Here's how the part is built. I have some questions about the finished solid (model axes, mm). A direction names the side the tool comes from. Coordinates: 2 decimals unless noted, no trailing zeros. Order: outer loops, then holes, each group sorted by start corner. A loop starts at its lowest first (then second) coordinate and runs counter-clockwise, first axis right, second up.
```python
from build123d import *

# Parameters (mm, degrees)
SKETCH_1_W                         = 1000
SKETCH_1_H                         = 368
SM_BASE_FLANGE_1_DEPTH             = 1
OTHER_START                        = -134.5
OTHER_1_DEPTH                      = 269
OTHER_1_2_DEPTH                    = 0.5
OTHER_START_2                      = 134
OTHER_1_3_DEPTH                    = 0.5
OTHER_START_3                      = -134
OTHER_1_4_DEPTH                    = 268
OTHER_START_4                      = -450.5
OTHER_2_DEPTH                      = 901
OTHER_2_2_DEPTH                    = 0.5
OTHER_START_5                      = 450
OTHER_2_3_DEPTH                    = 0.5
OTHER_START_6                      = -450
OTHER_2_4_DEPTH                    = 900
SM_EDGE_FLANGE_1_STRIP_W           = 5.4732
SM_EDGE_FLANGE_1_STRIP_H           = 1
SM_EDGE_FLANGE_1_STRIP_CUT_DEPTH   = 900
SM_EDGE_FLANGE_1_RELIEF_W          = 5.9732
SM_EDGE_FLANGE_1_RELIEF_H          = 0.5
SM_EDGE_FLANGE_1_RELIEF_CUT_DEPTH  = 1
SM_EDGE_FLANGE_1_DEPTH             = 900
SM_EDGE_FLANGE_1_FLAT_DEPTH        = 1
SM_EDGE_FLANGE_2_STRIP_W           = 5.4732
SM_EDGE_FLANGE_2_STRIP_H           = 1
SM_EDGE_FLANGE_2_STRIP_CUT_DEPTH   = 214.5
SM_EDGE_FLANGE_2_STRIP_2_W         = 5.4732
SM_EDGE_FLANGE_2_STRIP_2_H         = 1
SM_EDGE_FLANGE_2_STRIP_CUT_2_DEPTH = 412
SM_EDGE_FLANGE_2_STRIP_3_W         = 5.4732
SM_EDGE_FLANGE_2_STRIP_3_H         = 1
SM_EDGE_FLANGE_2_STRIP_CUT_3_DEPTH = 213.5
SM_EDGE_FLANGE_2_DEPTH             = 214.5
SM_EDGE_FLANGE_2_BEND_DEPTH        = 412
SM_EDGE_FLANGE_2_BEND_2_DEPTH      = 213.5
SKETCH_19_R                        = 3
CUT_EXTRUDE_1_DEPTH                = 534.120061525


# Read off the part's stored shape, not the designer's step: 斜接法兰1, 斜接法兰2
# Sheet-metal steps are written as plain solids
with BuildPart() as part:
    # Sketch 1 → 基体-法兰1 (new body)
    with BuildSketch(Plane.XY):
        Rectangle(SKETCH_1_W, SKETCH_1_H)
    extrude(amount=-SM_BASE_FLANGE_1_DEPTH)

    # Other 1 outline → Other 1 (cut)
    with BuildSketch(Plane(origin=(0, 0, 0), x_dir=(1, 0, 0), z_dir=(0, 1, 0)).offset(OTHER_START)):
        with BuildLine():
            Line((500, 1), (499.83604109, 1))
            ThreePointArc((499.83604109, 1), (499.195226164, 0.271171885), (498.2634, 0))
            Line((498.2634, 0), (500, 0))
            Line((500, 0), (500, 1))
        make_face()
    other_1 = extrude(amount=OTHER_1_DEPTH, mode=Mode.SUBTRACT)

    # Other 1 2 outline → Other 1 2 (cut)
    with BuildSketch(Plane(origin=(0, 0, 0), x_dir=(1, 0, 0), z_dir=(0, 1, 0)).offset(OTHER_START)):
        with BuildLine():
            ThreePointArc((498.2634, 0), (499.195226164, 0.271171885), (499.83604109, 1))
            Line((499.83604109, 1), (497.7634, 1))
            Line((497.7634, 1), (497.7634, 0))
            Line((497.7634, 0), (498.2634, 0))
        make_face()
    other_1_2 = extrude(amount=OTHER_1_2_DEPTH, mode=Mode.SUBTRACT)

    # Other 1 3 outline → Other 1 3 (cut)
    with BuildSketch(Plane(origin=(0, 0, 0), x_dir=(1, 0, 0), z_dir=(0, 1, 0)).offset(OTHER_START_2)):
        with BuildLine():
            ThreePointArc((498.2634, 0), (499.195226164, 0.271171885), (499.83604109, 1))
            Line((499.83604109, 1), (497.7634, 1))
            Line((497.7634, 1), (497.7634, 0))
            Line((497.7634, 0), (498.2634, 0))
        make_face()
    other_1_3 = extrude(amount=OTHER_1_3_DEPTH, mode=Mode.SUBTRACT)

    # Other 1 4 outline → Other 1 4 (add)
    with BuildSketch(Plane(origin=(0, 0, 0), x_dir=(1, 0, 0), z_dir=(0, 1, 0)).offset(OTHER_START_3)):
        with BuildLine():
            Line((500, 1.7366), (500, 18.2634))
            ThreePointArc((500, 18.2634), (499.491361636, 19.491361636), (498.2634, 20))
            Line((498.2634, 20), (485, 20))
            Line((485, 20), (485, 19))
            Line((485, 19), (498.2634, 19))
            ThreePointArc((498.2634, 19), (498.784254855, 18.784254855), (499, 18.2634))
            Line((499, 18.2634), (499, 1.7366))
            ThreePointArc((499, 1.7366), (498.784254855, 1.215745145), (498.2634, 1))
            Line((498.2634, 1), (499.83604109, 1))
            ThreePointArc((499.83604109, 1), (499.958514757, 1.359286442), (500, 1.7366))
        make_face()
    other_1_4 = extrude(amount=OTHER_1_4_DEPTH)

    # Other 2 outline → Other 2 (cut)
    with BuildSketch(Plane.YZ.offset(OTHER_START_4)):
        with BuildLine():
            ThreePointArc((182.2634, 0), (183.195226164, -0.271171885), (183.83604109, -1))
            Line((183.83604109, -1), (184, -1))
            Line((184, -1), (184, 0))
            Line((184, 0), (182.2634, 0))
        make_face()
    extrude(amount=OTHER_2_DEPTH, mode=Mode.SUBTRACT)

    # Other 2 2 outline → Other 2 2 (cut)
    with BuildSketch(Plane.YZ.offset(OTHER_START_4)):
        with BuildLine():
            Line((181.7634, -1), (183.83604109, -1))
            ThreePointArc((183.83604109, -1), (183.195226164, -0.271171885), (182.2634, 0))
            Line((182.2634, 0), (181.7634, 0))
            Line((181.7634, 0), (181.7634, -1))
        make_face()
    extrude(amount=OTHER_2_2_DEPTH, mode=Mode.SUBTRACT)

    # Other 2 3 outline → Other 2 3 (cut)
    with BuildSketch(Plane.YZ.offset(OTHER_START_5)):
        with BuildLine():
            Line((181.7634, -1), (183.83604109, -1))
            ThreePointArc((183.83604109, -1), (183.195226164, -0.271171885), (182.2634, 0))
            Line((182.2634, 0), (181.7634, 0))
            Line((181.7634, 0), (181.7634, -1))
        make_face()
    extrude(amount=OTHER_2_3_DEPTH, mode=Mode.SUBTRACT)

    # Other 2 4 outline → Other 2 4 (add)
    with BuildSketch(Plane.YZ.offset(OTHER_START_6)):
        with BuildLine():
            Line((184, -18.2634), (184, -1.7366))
            ThreePointArc((184, -1.7366), (183.958514757, -1.359286442), (183.83604109, -1))
            Line((183.83604109, -1), (182.2634, -1))
            ThreePointArc((182.2634, -1), (182.784254855, -1.215745145), (183, -1.7366))
            Line((183, -1.7366), (183, -18.2634))
            ThreePointArc((183, -18.2634), (182.784254855, -18.784254855), (182.2634, -19))
            Line((182.2634, -19), (169, -19))
            Line((169, -19), (169, -20))
            Line((169, -20), (182.2634, -20))
            ThreePointArc((182.2634, -20), (183.491361636, -19.491361636), (184, -18.2634))
        make_face()
    extrude(amount=OTHER_2_4_DEPTH)

    # 镜向1: Other 1, Other 1 2, Other 1 3, Other 1 4 across plane
    add(other_1.mirror(Plane(origin=(0, 0, 0), x_dir=(0, 0, 1), z_dir=(1, 0, 0))), mode=Mode.SUBTRACT)
    add(other_1_2.mirror(Plane(origin=(0, 0, 0), x_dir=(0, 0, 1), z_dir=(1, 0, 0))), mode=Mode.SUBTRACT)
    add(other_1_3.mirror(Plane(origin=(0, 0, 0), x_dir=(0, 0, 1), z_dir=(1, 0, 0))), mode=Mode.SUBTRACT)
    add(other_1_4.mirror(Plane(origin=(0, 0, 0), x_dir=(0, 0, 1), z_dir=(1, 0, 0))))

    # 边线-法兰1 strip (across the edge) → 边线-法兰1 strip cut (cut)
    with BuildSketch(Plane(origin=(450, -184, -1), x_dir=(0, 1, 0), z_dir=(-1, 0, 0))):
        with Locations((-1, -0.5)):
            Rectangle(SM_EDGE_FLANGE_1_STRIP_W, SM_EDGE_FLANGE_1_STRIP_H)
    extrude(amount=SM_EDGE_FLANGE_1_STRIP_CUT_DEPTH, mode=Mode.SUBTRACT)

    # 边线-法兰1 relief (on the sheet) → 边线-法兰1 relief cut (cut)
    with BuildSketch(Plane(origin=(450, -182.2634, -1), x_dir=(0, 1, 0), z_dir=(0, 0, -1))):
        with Locations((-2.4866, 0.25)):
            Rectangle(SM_EDGE_FLANGE_1_RELIEF_W, SM_EDGE_FLANGE_1_RELIEF_H)
        with Locations((-2.4866, -900.25)):
            Rectangle(SM_EDGE_FLANGE_1_RELIEF_W, SM_EDGE_FLANGE_1_RELIEF_H)
    extrude(amount=-SM_EDGE_FLANGE_1_RELIEF_CUT_DEPTH, mode=Mode.SUBTRACT)

    # 边线-法兰1 bend section (across the edge) → 边线-法兰1 (add)
    with BuildSketch(Plane(origin=(450, -184, -1), x_dir=(0, 1, 0), z_dir=(-1, 0, 0))):
        with BuildLine():
            Line((0, 0.7366), (1, 0.7366))
            ThreePointArc((1, 0.7366), (1.215745145, 0.215745145), (1.7366, 0))
            Line((1.7366, 0), (1.7366, -1))
            ThreePointArc((1.7366, -1), (0.508638364, -0.491361636), (0, 0.7366))
        make_face()
    extrude(amount=SM_EDGE_FLANGE_1_DEPTH)

    # 边线-法兰1 profile (on flange) → 边线-法兰1 flat (add)
    with BuildSketch(Plane(origin=(0, -184, -1), x_dir=(-1, 0, 0), z_dir=(0, -1, 0))):
        Polygon((-450, 0.7366), (450, 0.7366), (450, 19), (236.5, 19), (236.5, 1), (206.5, 1), (206.5, 19), (-205.5, 19), (-205.5, 1), (-235.5, 1), (-235.5, 19), (-450, 19), align=None)
    extrude(amount=-SM_EDGE_FLANGE_1_FLAT_DEPTH)

    # 边线-法兰2 strip (across the edge) → 边线-法兰2 strip cut (cut)
    with BuildSketch(Plane(origin=(450, -183, -20), x_dir=(0, 0, 1), z_dir=(-1, 0, 0))):
        with Locations((-1, -0.5)):
            Rectangle(SM_EDGE_FLANGE_2_STRIP_W, SM_EDGE_FLANGE_2_STRIP_H)
    extrude(amount=SM_EDGE_FLANGE_2_STRIP_CUT_DEPTH, mode=Mode.SUBTRACT)

    # 边线-法兰2 strip 2 (across the edge) → 边线-法兰2 strip cut 2 (cut)
    with BuildSketch(Plane(origin=(205.5, -183, -20), x_dir=(0, 0, 1), z_dir=(-1, 0, 0))):
        with Locations((-1, -0.5)):
            Rectangle(SM_EDGE_FLANGE_2_STRIP_2_W, SM_EDGE_FLANGE_2_STRIP_2_H)
    extrude(amount=SM_EDGE_FLANGE_2_STRIP_CUT_2_DEPTH, mode=Mode.SUBTRACT)

    # 边线-法兰2 strip 3 (across the edge) → 边线-法兰2 strip cut 3 (cut)
    with BuildSketch(Plane(origin=(-236.5, -183, -20), x_dir=(0, 0, 1), z_dir=(-1, 0, 0))):
        with Locations((-1, -0.5)):
            Rectangle(SM_EDGE_FLANGE_2_STRIP_3_W, SM_EDGE_FLANGE_2_STRIP_3_H)
    extrude(amount=SM_EDGE_FLANGE_2_STRIP_CUT_3_DEPTH, mode=Mode.SUBTRACT)

    # 边线-法兰2 section (across the edge) → 边线-法兰2 (add)
    with BuildSketch(Plane(origin=(450, -183, -20), x_dir=(0, 0, 1), z_dir=(-1, 0, 0))):
        with BuildLine():
            Line((0, 0.7366), (0, 14))
            Line((0, 14), (1, 14))
            Line((1, 14), (1, 0.7366))
            ThreePointArc((1, 0.7366), (1.215745145, 0.215745145), (1.7366, 0))
            Line((1.7366, 0), (1.7366, -1))
            ThreePointArc((1.7366, -1), (0.508638364, -0.491361636), (0, 0.7366))
        make_face()
    extrude(amount=SM_EDGE_FLANGE_2_DEPTH)

    # 边线-法兰2 section 2 (across the edge) → 边线-法兰2 bend (add)
    with BuildSketch(Plane(origin=(205.5, -183, -20), x_dir=(0, 0, 1), z_dir=(-1, 0, 0))):
        with BuildLine():
            Line((0, 0.7366), (0, 14))
            Line((0, 14), (1, 14))
            Line((1, 14), (1, 0.7366))
            ThreePointArc((1, 0.7366), (1.215745145, 0.215745145), (1.7366, 0))
            Line((1.7366, 0), (1.7366, -1))
            ThreePointArc((1.7366, -1), (0.508638364, -0.491361636), (0, 0.7366))
        make_face()
    extrude(amount=SM_EDGE_FLANGE_2_BEND_DEPTH)

    # 边线-法兰2 section 3 (across the edge) → 边线-法兰2 bend 2 (add)
    with BuildSketch(Plane(origin=(-236.5, -183, -20), x_dir=(0, 0, 1), z_dir=(-1, 0, 0))):
        with BuildLine():
            Line((0, 0.7366), (0, 14))
            Line((0, 14), (1, 14))
            Line((1, 14), (1, 0.7366))
            ThreePointArc((1, 0.7366), (1.215745145, 0.215745145), (1.7366, 0))
            Line((1.7366, 0), (1.7366, -1))
            ThreePointArc((1.7366, -1), (0.508638364, -0.491361636), (0, 0.7366))
        make_face()
    extrude(amount=SM_EDGE_FLANGE_2_BEND_2_DEPTH)

    # 草图19 → 切除-拉伸1 (cut, through all)
    with BuildSketch(Plane(origin=(0, 0, -1), x_dir=(-1, 0, 0), z_dir=(0, 0, -1))):
        with Locations((-491, 174)):
            Circle(SKETCH_19_R)
        with Locations((-491, -176)):
            Circle(SKETCH_19_R)
        with Locations((491, -176)):
            Circle(SKETCH_19_R)
        with Locations((491, 174)):
            Circle(SKETCH_19_R)
    extrude(amount=-CUT_EXTRUDE_1_DEPTH, mode=Mode.SUBTRACT)


solid = part.part
```
Q1. I need wall thicknesses on L1, parallel to X at y = -176, z = -0.4; L2, parallel to Y at x = -491, z = -0.7; L3, parallel to X at y = 28.5, z = -18.25. Which ranges of each line are inside material? Lowest first, please.
Q2. If we section it at A-A on z = -8.25: Write out the boundary of the cut face in (x, y).
Q3. If we section it at C-C on x = 56: Write out the boundary of the cut face in (y, z).
Q4. We'd pull the mould along Z, two halves only. Please class faces 1 (the flat face through (-7, 3, 0)), 2 (the flat face through (-6, 183, -10)), 3 (the flat face through (-499, -2, -10)), 4 (the flat face through (-500, -2, -10)): pulls with the +Z half, pulls with the -Z half, needs draft (parallel to the pull), parting line crosses it, or undercut.
Q5. If we section it at B-B on y = 25.5: Write out the boundary of the cut face in (x, z).
Q6. Will this pin go through, and if not, where does the flat tip stop? pin 1 (0.5 mm diameter, centred on y = -28.5, z = -19.5, fed in from -X).
Q7. For faces 5 (the flat face through (499, -2, -10)), 6 (the flat face through (6, -183, -10)), 7 (the flat face through (-6, 184, -10)), which set-ups out of +Z, -Z, +X, -X, +Y, -Y let a thin tool reach every point of the face, with its end or its side?
Reply:
1. L1: x = -500 to -494, -488 to 488, 494 to 500
1. L2: y = -184 to -179, -173 to 171, 177 to 184
1. L3: x = -500 to -499, 499 to 500
2. outline: (-500, -134) - (-499, -134) - (-499, 134) - (-500, 134) - close; (-450, -184) - (-236.5, -184) - (-236.5, -183) - (-450, -183) - close; (-450, 183) - (450, 183) - (450, 184) - (-450, 184) - close; (-206.5, -184) - (205.5, -184) - (205.5, -183) - (-206.5, -183) - close; (235.5, -184) - (450, -184) - (450, -183) - (235.5, -183) - close; (499, -134) - (500, -134) - (500, 134) - (499, 134) - close
3. outline: (-184, -18.26) arc R1.74 ccw to (-182.26, -20) - (-169, -20) - (-169, -19) - (-182.26, -19) arc R0.74 cw to (-183, -18.26) - (-183, -1.74) arc R0.74 cw to (-182.26, -1) - (182.26, -1) arc R0.74 cw to (183, -1.74) - (183, -18.26) arc R0.74 cw to (182.26, -19) - (169, -19) - (169, -20) - (182.26, -20) arc R1.74 ccw to (184, -18.26) - (184, -1.74) arc R1.74 ccw to (182.26, 0) - (-182.26, 0) arc R1.74 ccw to (-184, -1.74) - close
4. face 1: pulls with the +Z half
4. face 2: undercut
4. face 3: undercut
4. face 4: needs draft
5. outline: (-500, -18.26) arc R1.74 ccw to (-498.26, -20) - (-485, -20) - (-485, -19) - (-498.26, -19) arc R0.74 cw to (-499, -18.26) - (-499, -1.74) arc R0.74 cw to (-498.26, -1) - (498.26, -1) arc R0.74 cw to (499, -1.74) - (499, -18.26) arc R0.74 cw to (498.26, -19) - (485, -19) - (485, -20) - (498.26, -20) arc R1.74 ccw to (500, -18.26) - (500, -1.74) arc R1.74 ccw to (498.26, 0) - (-498.26, 0) arc R1.74 ccw to (-500, -1.74) - close
6. pin 1: stops at x = -499.69
7. face 5: +Y, -Y
7. face 6: +X, -X
7. face 7: +Z, -Z, +X, -X, +Y
